Check sheet for the modelled part. Datum: model origin and axes. Units: mm. Face numbers are marked on the shaded views. A direction names the side the tool comes from. Coordinates: 2 decimals unless noted, no trailing zeros. Loops run counter-clockwise (first coordinate to the right, second up) from the corner with the lowest first, then second, coordinate; pieces in that order, holes last. Notation, with made-up numbers: M -37.75,-37 L 11.25,-37 A9 ccw 11.25,-27 Z; hole C -4.5,-13 d7. An arc over 180 degrees is marked long. Write each question's results on one line, items separated by ' | '. Start each with the question number.
Autodesk Inventor part; units mm, degrees
ref_plane "YZ Plane" through (0, 0, 0) normal (1, 0, 0) x (0, 1, 0)
ref_plane "XZ Plane" through (0, 0, 0) normal (0, 1, 0) x (-1, 0, 0)
ref_plane "XY Plane" through (0, 0, 0) normal (0, 0, 1) x (1, 0, 0)
sketch "Sketch1" plane through (0, 0, 0) normal (0, 1, 0) x (-1, 0, 0)
  line L0 (0, 0) -> (11.2054, 0) construction
  line L1 (11.2054, 0) -> (0, 0) construction
  line L2 (-7.2218, -15) -> (-11.1109, -11.1109) construction
  line L3 (0, 0) -> (-11.1109, -11.1109) construction
  line L4 (-11.1109, -11.1109) -> (-7.2218, -15) construction
  line L5 (-11.1109, -18.8891) -> (0, -30) construction
  line L6 (-7.2218, -15) -> (-11.1109, -18.8891) construction
  line L7 (0, -30) -> (11.2054, -30) construction
  line L8 (11.2054, -30) -> (0, -30) construction
  line L9 (11.2054, -30) -> (11.2054, 0) construction
  line L10 (11.2054, 0) -> (11.2054, -30) construction
  line L11 (11.2054, 0) -> (11.2054, 1)
  line L12 (11.2054, 1) -> (0, 1)
  line L13 (0, 1) -> (-12.1109, -11.1109)
  line L14 (-12.1109, -11.1109) -> (-8.2218, -15)
  line L15 (-8.2218, -15) -> (-12.1109, -18.8891)
  line L16 (-12.1109, -18.8891) -> (0, -31)
  line L17 (0, -31) -> (11.2054, -31)
  line L18 (11.2054, -31) -> (11.2054, -30)
  line L19 (11.2054, -30) -> (0, -30)
  line L20 (-11.1109, -18.8891) -> (0, -30)
  line L21 (-11.1109, -18.8891) -> (-7.2218, -15)
  line L22 (-11.1109, -11.1109) -> (0, 0)
  line L23 (-11.1109, -11.1109) -> (-7.2218, -15)
  line L24 (11.2054, 0) -> (0, 0)
  point P0 (-20.2218, 0)
  dimension "d0" = 1
extrude "Extrusion1" add sketch "Sketch1" along normal blind 100
sketch "Sketch3" plane through (-11.2054, 0, 1) normal (0, 0, 1) x (1, 0, 0)
  line L0 (11.2053, -0.0014) -> (11.2053, 99.9986)
  line L1 (11.2053, 99.9986) -> (7.4271, 77.9986)
  circle A0 centre (7.4271, 74.9986) radius 3
  circle A1 centre (7.4271, 74.9986) radius 3
  line L2 (7.4271, 71.9986) -> (7.4271, 27.9986)
  circle A2 centre (7.4271, 24.9986) radius 3
  circle A3 centre (7.4271, 24.9986) radius 3
  point P0 (11.2054, 0)
  point P1 (0, 0)
extrude "Extrusion2" cut sketch "Sketch3" against normal up to surface (32 mm away)
properties part number "guardv2"
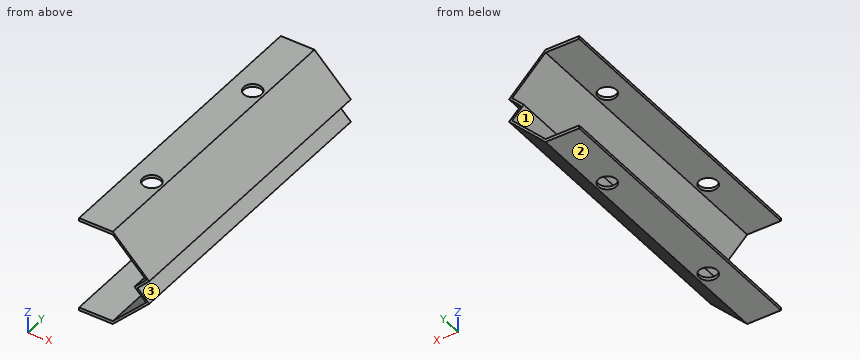
1) Section check D-D (z = -23). Enter the section's corners in (x, y), then the cut area to 3 significant figures.
2) Gauge pin test, flat ends, axial feed: P1, Ø4, axis at x = 6.5, y = 42.5, coming from the -Z side; P2, Ø1.5, axis at y = 49, z = -24, coming from the -X side; P3, Ø1, axis at y = 65, z = -12.5, coming from the -X side. Record the tip position at first contact, or that the pin passes through.
3) Set-up check for the marked faces 1, 2 and 3: record each of +Z, -Z, +X, -X, +Y, -Y from which the full face is reachable in a straight line by a thin tool's end or side.
4) Section check B-B (y = 87). Enter the section's corners in (x, z), then the cut area to 3 significant figures.
5) Thickness scan on probe 1 along Z at (x, y) = (-4, 67.5); probe 2 along Z at (x, y) = (7.5, 22.5); probe 3 along Z at (x, y) = (10, 4). Record the ranges inside material, lowest first.
6) Section check C-C (x = -1.75). Enter the section's corners in (y, z).
7) Section check A-A (x = 4.75). Enter the section's corners in (y, z), then the cut area to 3 significant figures.
Return value:
1) outline: M 7,0 L 8,0 L 8,100 L 7,100 Z | area: 100 mm2
2) P1: stops at z = -26.5 | P2: stops at x = 5.25 | P3: stops at x = 9.22
3) face 1: -X, +Y, -Y | face 2: -Z, +X, -X, +Y, -Y | face 3: +X, +Y, -Y
4) outline: M -11.21,-31 L 0,-31 L 12.11,-18.89 L 8.22,-15 L 12.11,-11.11 L 0,1 L -11.21,1 L -11.21,0 L 0,0 L 11.11,-11.11 L 7.22,-15 L 11.11,-18.89 L 0,-30 L -11.21,-30 Z | area: 53.4 mm2
5) probe 1: z = -31 to -30, 0 to 1 | probe 2: z = -23.5 to -22.5, -15.28 to -14.72, -7.5 to -6.5 | probe 3: z = -21 to -20, -17.78 to -16.78, -13.22 to -12.22, -10 to -9
6) outline: M 0,-31 L 22.79,-31 L 22.79,-30 L 0,-30 Z; M 0,0 L 22.79,0 L 22.79,1 L 0,1 Z; M 27.21,-31 L 72.79,-31 L 72.79,-30 L 27.21,-30 Z; M 27.21,0 L 72.79,0 L 72.79,1 L 27.21,1 Z; M 77.21,-31 L 100,-31 L 100,-30 L 77.21,-30 Z; M 77.21,0 L 100,0 L 100,1 L 77.21,1 Z
7) outline: M 0,-26.25 L 100,-26.25 L 100,-25.25 L 0,-25.25 Z; M 0,-4.75 L 100,-4.75 L 100,-3.75 L 0,-3.75 Z | area: 200 mm2
